Check sheet for the drawn part. Datum: minimum x, y, z corner. Units: mm. A direction names the side the tool comes from. Round coordinates to 2 decimals unless told otherwise and drop trailing zeros. Write each loop counter-clockwise with the first axis right and the second up, starting at its lowest first coordinate (ties: lowest second). Pieces come first, ordered by that corner, then holes. Notation, with made-up numbers: M 85.5,9 L 135.5,9 A16 ccw 135.5,21 Z; hole C 74.25,-39.5 d7. An arc over 180 degrees is marked long. Put each result on its own line as item: value.
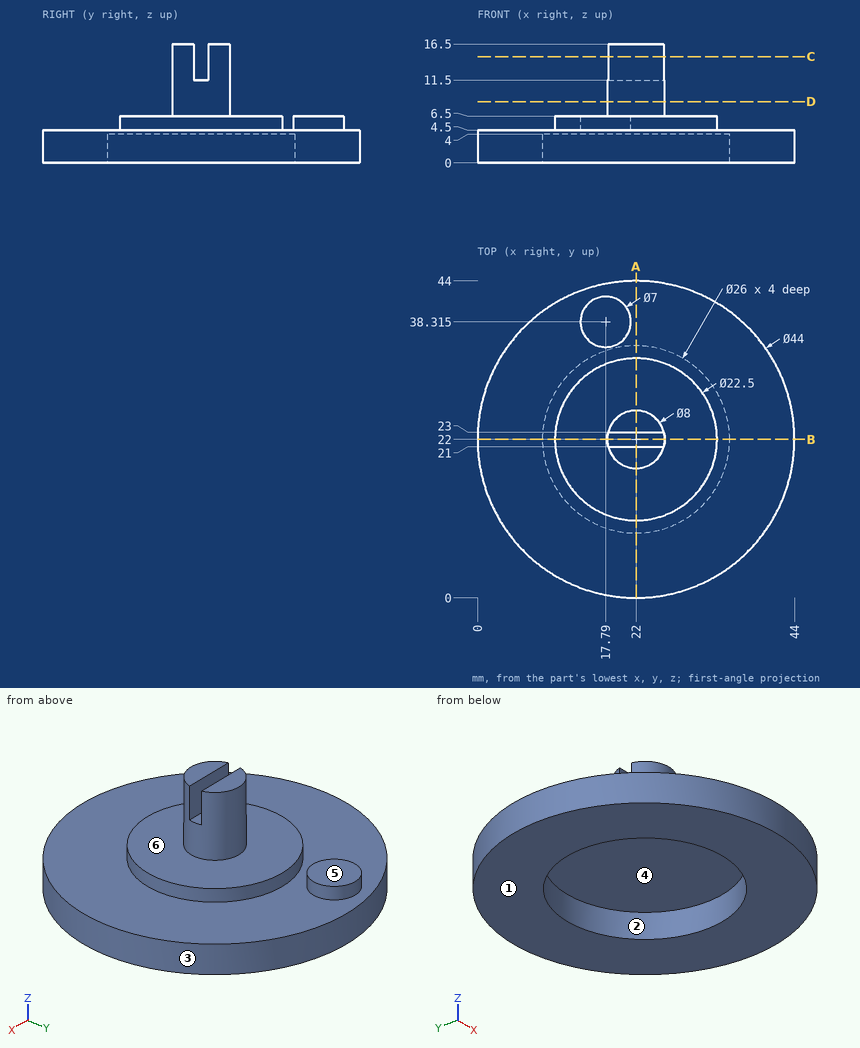
1. Cross-section at C-C (z = 14.75). Enter the section's corners in (x, y).
Computed values:
outline: M 18.13,21 A4 ccw 25.87,21 Z; M 18.13,23 L 25.87,23 A4 ccw Z
2. Cross-section at B-B (y = 22). Enter the section's corners in (x, z).
Computed values:
outline: M 0,0 L 9,0 L 9,4 L 35,4 L 35,0 L 44,0 L 44,4.5 L 33.25,4.5 L 33.25,6.5 L 26,6.5 L 26,11.5 L 18,11.5 L 18,6.5 L 10.75,6.5 L 10.75,4.5 L 0,4.5 Z
3. Depth check by flat-ended pin: pin 1 Ø8 at (y, z) = (15, 3.5) entering from -X (1 decimal); pin 2 Ø5.5 at (x, z) = (21, 13.5) entering from -Y; pin 3 Ø2 at (y, z) = (19.5, 11.5) entering from +X. Enter the tip coordinate at first touch or a pass-through.
Computed values:
pin 1: stops at x = 0.2
pin 2: stops at y = 18
pin 3: stops at x = 25.71
4. Cross-section at A-A (x = 22). Enter the section's corners in (y, z).
Computed values:
outline: M 0,0 L 9,0 L 9,4 L 35,4 L 35,0 L 44,0 L 44,4.5 L 33.25,4.5 L 33.25,6.5 L 26,6.5 L 26,16.5 L 23,16.5 L 23,11.5 L 21,11.5 L 21,16.5 L 18,16.5 L 18,6.5 L 10.75,6.5 L 10.75,4.5 L 0,4.5 Z
5. Release check for a two-part mould opening along X. For the marked faces 1, 2 and 3 record: +X half, -X half, draft (parallel to the pull), parting line (faces both ways), or undercut.
Computed values:
face 1: draft
face 2: undercut
face 3: parting line
6. Cross-section at D-D (z = 8.5). Enter the section's corners in (x, y).
Computed values:
outline: C 22,22 d8
7. Access from +Z, -Z, +X, -X, +Y, -Y to the whole of each face (thin tool, end or side, straight path). Record for the marked faces 4, 5 and 6.
Computed values:
face 4: -Z
face 5: +Z, +X, -X, +Y
face 6: +Z
8. Scan lines: probe 1 along Y at (x, z) = (22, 1.35); probe 2 along Z at (x, y) = (34.5, 27); probe 3 along Y at (x, z) = (22.5, 4.75). Record each from-to range of solid material in increasing order.
Computed values:
probe 1: y = 0 to 9, 35 to 44
probe 2: z = 0 to 4.5
probe 3: y = 10.76 to 33.24
